```python
from build123d import *

# Parameters (mm, degrees)
TUBE_R            = 5.2
TUBE_R_2          = 2.5
TUBE_DEPTH        = 3.9
CYLINDER001_R     = 2.65
CYLINDER001_DEPTH = 15
CYLINDER005_R     = 7.5
CYLINDER005_DEPTH = 8


with BuildPart() as lower_shaft_bearing:
    # Tube → Tube (new body)
    with BuildSketch(Plane.XY.offset(9)):
        Circle(TUBE_R)
        Circle(TUBE_R_2, mode=Mode.SUBTRACT)
    extrude(amount=TUBE_DEPTH)


with BuildPart() as lower_shaft_bearing_1:
    # BaseFeature004 placement: moved
    add(lower_shaft_bearing.part.moved(Location((0, 0, -9))))


with BuildPart() as lower_shaft_bearing_2:
    # Body038 placement: moved
    add(lower_shaft_bearing_1.part.moved(Location((0, 0, 9))))


with BuildPart() as fusion001:
    # Cylinder001 → Cylinder001 (new body)
    with BuildSketch(Plane.XY.offset(1.5)):
        Circle(CYLINDER001_R)
    extrude(amount=CYLINDER001_DEPTH)


with BuildPart() as fusion001_1:
    # BaseFeature003 placement: moved
    add(fusion001.part.moved(Location((0, 0, -1.5))))


with BuildPart() as fusion001_2:
    # Body014 placement: moved
    add(fusion001_1.part.moved(Location((0, 0, 1.5))))

    # Fusion001: union lower_shaft_bearing
    add(lower_shaft_bearing_2.part)


with BuildPart() as cut002:
    # Cylinder005 → Cylinder005 (join)
    with BuildSketch(Plane.XY):
        Circle(CYLINDER005_R)
    extrude(amount=CYLINDER005_DEPTH)


with BuildPart() as cut002_1:
    # Body019 placement: moved
    add(cut002.part.moved(Location((0, 0, 10))))

    # Cut002: cut Fusion001
    add(fusion001_2.part, mode=Mode.SUBTRACT)


solid = cut002_1.part
```
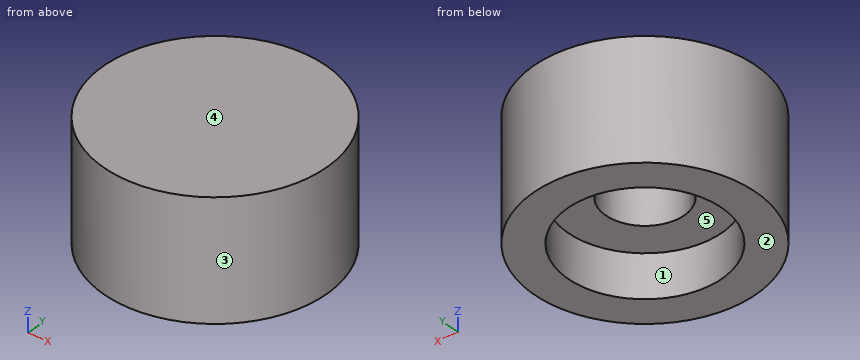
Build history of the part. All positions in model axes, mm. Face numbers are marked on the shaded views. A direction names the side the tool comes from. Round coordinates to 2 decimals unless told otherwise and drop trailing zeros. Write each loop counter-clockwise with the first axis right and the second up, starting at its lowest first coordinate (ties: lowest second). Pieces come first, ordered by that corner, then holes. Notation, with made-up numbers: (79.25, 25.25) -> (121.25, 25.25) arc R12 cw to (121.25, 40.25) -> close; hole circle Ø8 at (64.25, 11). An arc over 180 degrees is marked (long way). Put each result on its own line as item: value.
Item 1: Slice it at A-A, the plane x = 0. Give the cut face in (y, z).
Here are the results:
outline: (-7.5, 10) -> (-5.2, 10) -> (-5.2, 12.9) -> (-2.65, 12.9) -> (-2.65, 16.5) -> (2.65, 16.5) -> (2.65, 12.9) -> (5.2, 12.9) -> (5.2, 10) -> (7.5, 10) -> (7.5, 18) -> (-7.5, 18) -> close
Item 2: Tool access for the marked faces 4 and 5: list every direction of +Z, -Z, +X, -X, +Y, -Y with a clear straight run to the whole face (end or side of a thin tool).
Here are the results:
face 4: +Z, +X, -X, +Y, -Y
face 5: -Z
Item 3: Slice it at C-C, the plane z = 12. Give the cut face in (x, y), plus the area to 3 significant figures.
Here are the results:
outline: circle Ø15 at (0, 0); hole circle Ø10.4 at (0, 0)
area: 91.8 mm^2
Item 4: Two-plate mould, pull along X, no slides. Class the marked faces 1, 2 and 3: pulls with the +X half, pulls with the -X half, needs draft (parallel to the pull), parting line crosses it, or undercut.
Here are the results:
face 1: undercut
face 2: needs draft
face 3: parting line crosses it
Item 5: Slice it at D-D, the plane x = 4.75. Give the cut face in (y, z).
Here are the results:
outline: (-5.8, 10) -> (-2.12, 10) -> (-2.12, 12.9) -> (2.12, 12.9) -> (2.12, 10) -> (5.8, 10) -> (5.8, 18) -> (-5.8, 18) -> close
Item 6: Flat gauge pins, fed straight in: P1, Ø4, axis at x = 0.5, y = 0, coming from the -Z side; P2, Ø8.5, axis at x = 0, y = 0, coming from the -Z side. Where does each tip first touch, or does it go through?
Here are the results:
P1: stops at z = 16.5
P2: stops at z = 12.9
Item 7: Wall check: probe 1 along Y at (x, z) = (0, 11.65); probe 2 along Y at (x, z) = (0, 14.35); probe 3 along Z at (x, y) = (-0.75, 0.5). Give the ranges that are in metal, low to high. Write a range as from..to.
Here are the results:
probe 1: y = -7.5..-5.2, 5.2..7.5
probe 2: y = -7.5..-2.65, 2.65..7.5
probe 3: z = 16.5..18
